Autodesk Inventor part; units mm, degrees
ref_plane "YZ Plane" through (0, 0, 0) normal (1, 0, 0) x (0, 1, 0)
ref_plane "XZ Plane" through (0, 0, 0) normal (0, 1, 0) x (-1, 0, 0)
ref_plane "XY Plane" through (0, 0, 0) normal (0, 0, 1) x (1, 0, 0)
sketch "Sketch1" plane through (0, 0, 0) normal (0, 1, 0) x (-1, 0, 0)
  line L0 (10, 25) -> (-10, 25)
  line L1 (-10, 25) -> (-10, -25)
  line L2 (-10, -25) -> (10, -25)
  line L3 (10, -25) -> (10, 25)
  point P0 (0, 0)
  point P1 (0, -25)
  point P2 (10, 0)
  dimension "d0" = 20
  dimension "d1" = 50
extrude "Extrusion1" add sketch "Sketch1" along normal blind 3
sketch "Sketch2" plane through (0, 3, 0) normal (0, 1, 0) x (1, 0, 0)
  line L0 (-10, -25) -> (10, -25)
  point P0 (0, 0)
  point P1 (0, -17.5)
  point P2 (0, -2.5)
  dimension "d4" = 15
  dimension "d6" = 7.5
hole "Hole1" at (0, 3, 17.5) at (0, 3, 2.5) direction (0, -1, 0) diameter 4.5 end through all
properties part number "Endstop Mounting Plate"
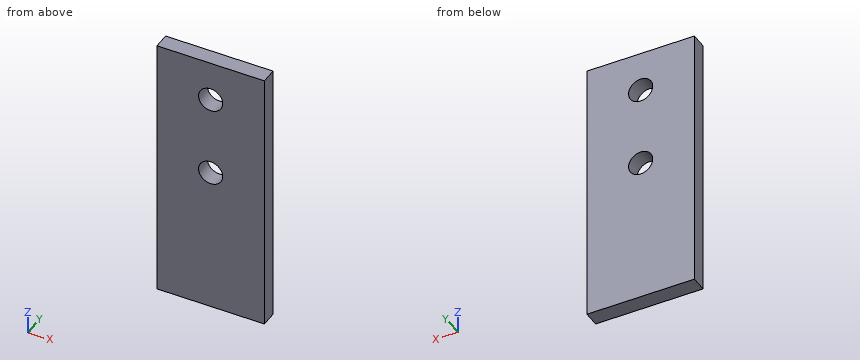
Here's how the part is built. I have some questions about the finished solid (model axes, mm). Round coordinates to 2 decimals unless told otherwise and drop trailing zeros. Write each loop counter-clockwise with the first axis right and the second up, starting at its lowest first coordinate (ties: lowest second). Pieces come first, ordered by that corner, then holes. Notation, with made-up numbers: M 83.5,72 L 102.5,72 A15 ccw 102.5,95 Z; hole C -27.75,22.5 d11. An arc over 180 degrees is marked long. Answer as CSV lines item,"result". Start each with the question number.
1. I'm going to push flat-ended pins straight in: pin 1 Ø2.5 at (x, z) = (0, 2.5) entering from -Y; pin 2 Ø8 at (x, z) = (-5.5, 15.5) entering from -Y. Where does each tip first touch, or does it pass through?
2. Suppose I cut it at C-C on y = 1.25. Write out the boundary of the cut face in (x, z).
3. Suppose I cut it at B-B on x = 0. Write out the boundary of the cut face in (y, z).
4. I need wall thicknesses on probe 1 along Z at (x, y) = (0, 2.1); probe 2 along X at (y, z) = (2.1, 2.5); probe 3 along Z at (x, y) = (-1.25, 1.35). Which ranges of each line are inside material? Lowest first, please.
5. Suppose I cut it at A-A on z = 2.5. Write out the boundary of the cut face in (x, y).
Check result:
1,pin 1,"passes through"
1,pin 2,"stops at y = 0"
2,outline,"M -10,-25 L 10,-25 L 10,25 L -10,25 Z; hole C 0,2.5 d4.5; hole C 0,17.5 d4.5"
3,outline,"M 0,-25 L 3,-25 L 3,0.25 L 0,0.25 Z; M 0,4.75 L 3,4.75 L 3,15.25 L 0,15.25 Z; M 0,19.75 L 3,19.75 L 3,25 L 0,25 Z"
4,probe 1,"z = -25 to 0.25, 4.75 to 15.25, 19.75 to 25"
4,probe 2,"x = -10 to -2.25, 2.25 to 10"
4,probe 3,"z = -25 to 0.63, 4.37 to 15.63, 19.37 to 25"
5,outline,"M -10,0 L -2.25,0 L -2.25,3 L -10,3 Z; M 2.25,0 L 10,0 L 10,3 L 2.25,3 Z"
